from build123d import *

# Parameters (mm, degrees)
F2_R     = 0.2
F3_W     = 35.523725
F3_H     = 30.81022
F4_DEPTH = 25


with BuildPart() as f1:
    # F0 (on Front) → F1 (revolve)
    with BuildSketch(Plane.XZ):
        with BuildLine():
            Line((6.5, 2.283427), (3, 2.283427))
            Line((3, 2.283427), (3, -3.716573))
            Line((3, -3.716573), (3.75, -3.716573))
            Line((3.75, -3.716573), (3.75, -1.716573))
            ThreePointArc((3.75, -1.716573), (4.75, -0.716573), (5.75, -1.716573))
            Line((5.75, -1.716573), (5.75, -3.716573))
            Line((5.75, -3.716573), (6.5, -3.716573))
            Line((6.5, -3.716573), (6.5, 2.283427))
        make_face()
    revolve(axis=Axis((0, 0, -0.059434), (0, 0, -1)))

    # F2
    f2_edges = [f1.edges().sort_by_distance(p)[0] for p in [
        (-5.75, 0, -3.716573),
        (-3.75, 0, -3.716573),
    ]]
    fillet(f2_edges, radius=F2_R)

    # F3 (on Front) → F4 (cut)
    with BuildSketch(Plane.XZ):
        with Locations((2.952699, 0.107419)):
            Rectangle(F3_W, F3_H)
    extrude(amount=-F4_DEPTH, mode=Mode.SUBTRACT)


solid = f1.part
Can you work these out from the model? Positions are in its coordinate system, mm. Give positions to 0.01 mm unless a question says otherwise; leave off trailing zeros. Loops run counter-clockwise (first coordinate to the right, second up) from the corner with the lowest first, then second, coordinate; pieces in that order, holes last. Notation, with made-up numbers: (36, -2) - (59, -2) arc R38 cw to (59, 37) - close; hole circle Ø3 at (68, 1). An arc over 180 degrees is marked (long way). Return JSON: item names as keys, results as strings.
1. I want a section at B-B on z = 1.25. Please give me the cut outline in (x, y).
Output values:
{"outline": "(-6.5, 0) arc R6.5 ccw to (6.5, 0) - (3, 0) arc R3 cw to (-3, 0) - close"}
2. I want a section at A-A on x = 0. Please give me the cut outline in (y, z), and give its area (3 significant figures).
Output values:
{"outline": "(-6.5, -3.72) - (-5.95, -3.72) arc R0.2 ccw to (-5.75, -3.52) - (-5.75, -1.72) arc R1 cw to (-3.75, -1.72) - (-3.75, -3.52) arc R0.2 ccw to (-3.55, -3.72) - (-3, -3.72) - (-3, 2.28) - (-6.5, 2.28) - close", "area": "15.4 mm²"}
3. I'm going to push flat-ended pins straight in: pin 1 Ø1 at (y, z) = (-5, -2.5) entering from +X; pin 2 Ø1 at (y, z) = (-4.5, -2.5) entering from -X; pin 3 Ø1 at (y, z) = (-2, -3) entering from +X. Where does each tip first touch, or does it pass through?
Output values:
{"pin 1": "stops at x = 4.69", "pin 2": "stops at x = -5.12", "pin 3": "stops at x = 6.32"}
4. If I drill on line 1 (X direction, y = -1.25, z = 2.25); line 2 (X direction, y = -4.5, z = -3); line 3 (X direction, y = -1.5, z = -1.75), over which ranges is the centre line in solid material (lowest first)?
Output values:
{"line 1": "x = -6.38 to -2.73, 2.73 to 6.38", "line 2": "x = -4.69 to -3.58, 3.58 to 4.69", "line 3": "x = -6.32 to -5.55, -3.44 to -2.6, 2.6 to 3.44, 5.55 to 6.32"}
5. We'd pull the mould along X, two halves only. Please class faces 1 (the face through (5, 0, 0)), 2 (the face through (0.1, -6.5, -0.7)), 3 (the face through (0.13, -5.75, -2.63)), 4 (the face through (0.08, -3.75, -2.6)): +X half, -X half, draft (parallel to the pull), parting line (faces both ways), or undercut.
Output values:
{"face 1": "draft", "face 2": "parting line", "face 3": "undercut", "face 4": "undercut"}
